Here's how the part is built. I have some questions about the finished solid (model axes, mm). A direction names the side the tool comes from. Coordinates: 2 decimals unless noted, no trailing zeros. Order: outer loops, then holes, each group sorted by start corner. A loop starts at its lowest first (then second) coordinate and runs counter-clockwise, first axis right, second up. Notation, with made-up numbers: (52.5, -30.5) - (104.5, -30.5) arc R20 cw to (104.5, -8.5) - close; hole circle Ø9 at (-29, -35). An arc over 180 degrees is marked (long way). Answer as CSV lines item,"result". Start each with the question number.
Q1. I need wall thicknesses on line 1 (Z direction, x = -4.4, y = -13.9); line 2 (Z direction, x = -3.5, y = -18.15); line 3 (Y direction, x = -1, z = -3.5). Which ranges of each line are inside material? Lowest first, please.
Q2. For pin 1 Ø4 at (x, z) = (2.5, -6.5) entering from -Y; pin 2 Ø0.6 at (x, y) = (7, -14.5) entering from +Z; pin 3 Ø1.7 at (y, z) = (-16.5, 3.5) entering from +X, each with a flat end and sliding along its axis, tell me the tip position at first contact or that it passes through.
Q3. Suppose I cut it at A-A (z = -9.7). Please give me the cut outline in (x, y), then the cut area to 4 significant figures.
Q4. Suppose I cut it at B-B (x = -5). Please give me the cut outline in (y, z), then the cut area to 3 significant figures.
Q5. Suppose I cut it at D-D (x = -0.25). Please give me the cut outline in (y, z), then the cut area to 3 significant figures.
Q6. For faces 1 (the face through (6.5, -16, 5)), 2 (the face through (-3.51, -14.26, -8.31)), 3 (the face through (0, -15, -7)), 4 (the face through (-0.76, -15.47, 9.54)), 5 (the face through (0, -14, -16.2)), which set-ups out of +Z, -Z, +X, -X, +Y, -Y let a thin tool reach every point of the face, with its end or its side?
Q7. Thinking about a two-plate mould opening in Z: for faces 6 (the face through (0, -17, 1.8)), 7 (the face through (-7, -14, -7)), 8 (the face through (-6.5, -16, 5)), which applies, released by +Z, released by -Z, zero draft, split by the parting line, or undercut?
Q8. Suppose I cut it at C-C (y = -16.2). Please give me the cut outline in (x, z).
from build123d import *

# Parameters (mm, degrees)
F0_W     = 14
F0_H     = 18
F1_DEPTH = 1.5
F2_W     = 13
F2_H     = 6
F3_DEPTH = 5.75
F4_R     = 1.65
F5_DEPTH = 25
F7_DEPTH = 4
F8_ANGLE = -90


with BuildPart() as f1:
    # F0 (on Top) → F1 (new body)
    with BuildSketch(Plane.XY):
        Rectangle(F0_W, F0_H)
    extrude(amount=F1_DEPTH)

    # F2 (on Top) → F3 (join)
    with BuildSketch(Plane.XY):
        with Locations((0, 12)):
            Rectangle(F2_W, F2_H)
    extrude(amount=F3_DEPTH)

    # F4 (on face) → F5 (cut)
    with BuildSketch(Plane.XY.offset(1.5)):
        with Locations((-4.4, -2.5)):
            Circle(F4_R)
    extrude(amount=-F5_DEPTH, mode=Mode.SUBTRACT)

    # F6 (on Top) → F7 (join)
    with BuildSketch(Plane.XY):
        Polygon((5.727259339, 15), (6.5, 15), (-7.022961568, 18.6234666314), (-7.0747253771, 18.4302814662), align=None)
    extrude(amount=F7_DEPTH)


with BuildPart() as f1_1:
    # F8: moved
    add(f1.part.rotate(Axis((0, -9, 1.5), (-1, 0, 0)), F8_ANGLE))


with BuildPart() as f1_2:
    # F9: moved
    add(f1_1.part.moved(Location((0, -6, -17.7))))


solid = f1_2.part
Here are the results:
1,line 1,"z = -16.2 to -11.35, -8.05 to 7.8, 10.51 to 10.72"
1,line 2,"z = 1.8 to 7.8"
1,line 3,"y = -15 to -13.5"
2,pin 1,"stops at y = -15"
2,pin 2,"stops at z = 1.8"
2,pin 3,"stops at x = 6.5"
3,outline,"(-7, -15) - (-6.05, -15) - (-6.05, -13.5) - (-7, -13.5) - close; (-2.75, -15) - (7, -15) - (7, -13.5) - (-2.75, -13.5) - close"
3,area,"16.05 mm²"
4,outline,"(-19.25, 1.8) - (-15, 1.8) - (-15, -8.16) - (-13.5, -8.16) - (-13.5, 7.8) - (-19.25, 7.8) - close; (-17.5, 10.67) - (-13.5, 10.67) - (-13.5, 10.88) - (-17.5, 10.88) - close; (-15, -16.2) - (-13.5, -16.2) - (-13.5, -11.24) - (-15, -11.24) - close"
4,area,"57.7 mm²"
5,outline,"(-19.25, 1.8) - (-15, 1.8) - (-15, -16.2) - (-13.5, -16.2) - (-13.5, 7.8) - (-19.25, 7.8) - close; (-17.5, 9.4) - (-13.5, 9.4) - (-13.5, 9.61) - (-17.5, 9.61) - close"
5,area,"62.3 mm²"
6,face 1,"+Z, +X, +Y, -Y"
6,face 2,"+Y, -Y"
6,face 3,"-Z, +X, -X, -Y"
6,face 4,"-X, +Y, -Y"
6,face 5,"-Z, +X, -X, +Y, -Y"
7,face 6,"released by -Z"
7,face 7,"zero draft"
7,face 8,"undercut"
8,outline,"(-7.07, 11.23) - (5.73, 7.8) - (-6.5, 7.8) - (-6.5, 1.8) - (6.5, 1.8) - (6.5, 7.8) - (-7.02, 11.42) - close"
